Design review of the part built by this model. Coordinates are the model's own, in mm. Face numbers are marked on the shaded views. A direction names the side the tool comes from. Give positions to 0.01 mm unless a question says otherwise; leave off trailing zeros. Write each loop counter-clockwise with the first axis right and the second up, starting at its lowest first coordinate (ties: lowest second). Pieces come first, ordered by that corner, then holes. Notation, with made-up numbers: M -23,-36.5 L 18,-36.5 A16 ccw 18,-28.5 Z; hole C 58,46.25 d9. An arc over 180 degrees is marked long. One line per item, written item: value. Start each with the question number.
```python
from build123d import *

# Parameters (mm, degrees)
F0_W     = 35.3952348232
F0_H     = 27.7462676167
F1_DEPTH = 155.0669968128
F3_DEPTH = 155.3752869368
F4_DEPTH = 14.4026782364


with BuildPart() as f1:
    # F0 (on Front) → F1 (new body)
    with BuildSketch(Plane.XZ):
        with Locations((1.4998167753, 27.5213085115)):
            Rectangle(F0_W, F0_H)
    extrude(amount=F1_DEPTH)

    # F2 (on face) → F3 (join)
    with BuildSketch(Plane.XZ.offset(155.0669968128)):
        with BuildLine():
            ThreePointArc((19.1974341869, 16.066663446), (23.0552776861, 20.5771904827), (24.4421993637, 26.3481747031))
            ThreePointArc((24.4421993637, 26.3481747031), (23.0552776861, 32.1191589236), (19.1974341869, 36.6296859603))
            Line((19.1974341869, 36.6296859603), (19.1974341869, 16.066663446))
        make_face()
    extrude(amount=-F3_DEPTH)

    # F4 (add): faces of the model
    f4_faces = [f1.faces().sort_by_distance(p)[0] for p in [
        (1.4998167753, 0, 27.5213085115),
        (21.3375597344, 0.3082901239, 26.3481747031),
    ]]
    extrude(f4_faces, amount=F4_DEPTH)


solid = f1.part
```
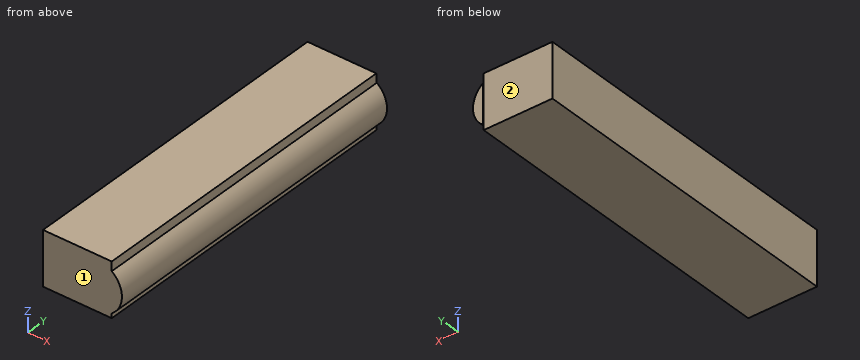
Q1. Take a section at C-C, the plane x = 21. Give the boundary of the cut face in (y, z), then the cut area to 3 significant figures.
Q2. Take a section at A-A, the plane y = -141. Give the boundary of the cut face in (x, z).
Q3. Take a section at B-B, the plane z = 31. Give the boundary of the cut face in (x, y).
Q4. For P1, Ø10, axis at y = -84, z = 24.5, coming from the +X side; P2, Ø2.5, axis at y = -107.5, z = 15.5, coming from the +X side; P3, Ø8.5, axis at x = 1, z = 30.5, coming from the +Y side; P4, Ø2.5, axis at y = -42, z = 40, coming from the +X side, all flat-tipped, find the tip position at first contact; note any pin that passes through.
Q5. Machinability: for the marked faces 1 and 2, which of the approach directions +Z, -Z, +X, -X, +Y, -Y give a long, thin tool a straight path to every point of the face, cutting with its end or side? Answer none if there is none.
Q6. Wall thickness on line 1 (Y direction, x = 8.5, z = 24.5); line 2 (X direction, y = -26, z = 15); line 3 (X direction, y = -143.5, z = 22.5): over which ranges is each line inside the solid? List them lowest first. Write a range as from..to.
Results list:
1. outline: M -155.07,17.65 L 14.71,17.65 L 14.71,35.04 L -155.07,35.04 Z
1. area: 2,950 mm^2
2. outline: M -16.2,13.65 L 19.2,13.65 L 19.2,16.07 A12.7 ccw 19.2,36.63 L 19.2,41.39 L -16.2,41.39 Z
3. outline: M -16.2,-155.07 L 23.56,-155.07 L 23.56,14.71 L 19.2,14.71 L 19.2,14.4 L -16.2,14.4 Z
4. P1: stops at x = 24.44
4. P2: stops at x = 20.06
4. P3: stops at y = 14.4
4. P4: stops at x = 19.2
5. face 1: +Z, -Z, +X, -X, -Y
5. face 2: +Z, -Z, -X, +Y
6. line 1: y = -155.07..14.4
6. line 2: x = -16.2..19.2
6. line 3: x = -16.2..23.85
